The model under review builds one solid part; all positions refer to its coordinate system, in mm. A direction names the side the tool comes from. Round coordinates to 2 decimals unless told otherwise and drop trailing zeros. Write each loop counter-clockwise with the first axis right and the second up, starting at its lowest first coordinate (ties: lowest second). Pieces come first, ordered by that corner, then holes. Notation, with made-up numbers: M 33,69.5 L 79,69.5 A37 cw 79,107.5 Z; hole C -28.75,5.25 d8. An arc over 180 degrees is marked long. One line per item, written item: value. Start each with the question number.
1) Take a section at D-D, the plane x = -89. Write out the cut boundary in (y, z).
2) Take a section at C-C, the plane z = -23. Write out the cut boundary in (x, y), and give its area (3 significant figures).
3) Tool access review of faces 1 (the face through (-23.846, -107.384, -18.734)), 2 (the face through (93.2, -59.1, 25)), 3 (the face through (60, -60, 22)): name each direction out of +Z, -Z, +X, -X, +Y, -Y from which nothing blocks a thin tool from reaching the whole face with its end or side.
4) For P1, Ø6, axis at x = -78, y = -67.5, coming from the -Z side; P2, Ø2, axis at x = -14.5, z = 17, coming from the -Y side; P3, Ø6, axis at x = 50, z = 2.5, coming from the +Y side, all flat-tipped, find the tip position at first contact; note any pin that passes through.
5) Take a section at A-A, the plane x = 0. Write out the cut boundary in (y, z).
6) Mouldability with a two-part tool opening along Y and no side actions: class faces 4 (the face through (-24.93, -112.265, -6.941)), 5 (the face through (-60, 60, 22)), 6 (the face through (0, 0, -38)) as +Y half, -Y half, draft (parallel to the pull), parting line (faces both ways), or undercut.
7) Wall thickness on probe 1 along Y at (x, z) = (13.5, -15.5); probe 2 along Y at (x, z) = (0, 21.75): over which ranges is each line inside the solid? List them lowest first.
from build123d import *

# Parameters (mm, degrees)
F0_R           = 115
F1_DEPTH       = 15
F2_R           = 17.5
F3_DEPTH       = 38
F4_R           = 17.5
F5_DEPTH       = 7
F6_R           = 15.5
F7_DEPTH       = 15.5
F8_R           = 15.49999
F10_R          = 115
F10_R_2        = 110
F11_DEPTH      = 10
F11_DEPTH_BACK = 53


# Not quite as in the source:
# - a fillet or chamfer that OpenCascade refuses, or shapes differently, is made with other operations: its cross-section is extruded or revolved along the edge and cut away or added
# - a fillet or chamfer is up to 0.001 mm smaller than in the source, because OpenCascade refuses the exact size


with BuildPart() as f1:
    # F0 (on Top) → F1 (new body)
    with BuildSketch(Plane.XY):
        Circle(F0_R)
    extrude(amount=F1_DEPTH)

    # F2 (on face) → F3 (join)
    with BuildSketch(Plane(origin=(0, 0, 0), x_dir=(1, 0, 0), z_dir=(0, 0, -1))):
        Circle(F2_R)
    extrude(amount=F3_DEPTH)

    # F4 (on face) → F5 (join)
    with BuildSketch(Plane.XY.offset(15)):
        with Locations((-60, 60)):
            Circle(F4_R)
        with Locations((-60, -60)):
            Circle(F4_R)
        with Locations((60, -60)):
            Circle(F4_R)
        with Locations((60, 60)):
            Circle(F4_R)
    extrude(amount=F5_DEPTH)

    # F6 (on face) → F7 (cut)
    with BuildSketch(Plane(origin=(0, 0, 0), x_dir=(1, 0, 0), z_dir=(0, 0, -1))):
        with Locations((-60, 60)):
            Circle(F6_R)
        with Locations((-60, -60)):
            Circle(F6_R)
        with Locations((60, -60)):
            Circle(F6_R)
        with Locations((60, 60)):
            Circle(F6_R)
    extrude(amount=-F7_DEPTH, mode=Mode.SUBTRACT)

    # F8 (radius 15.5 in the source; OpenCascade refuses exactly that, so slightly less here)
    f8_edges = [f1.edges().sort_by_distance(p)[0] for p in [
        (-75.5, -60, 15.5),
        (44.5, -60, 15.5),
        (44.5, 60, 15.5),
        (-75.5, 60, 15.5),
    ]]
    fillet(f8_edges, radius=F8_R)

    # F9: fillet of radius 12 on 4 edges, made by hand

    # F9_s1 → F9_t2 (revolve, cut)
    with BuildSketch(Plane.XZ.offset(60)):
        with BuildLine():
            ThreePointArc((-42.5, 15), (-46.9279714162, 20.0995049384), (-53.4087121146, 22))
            Line((-53.4087121146, 22), (-42.5, 22))
            Line((-42.5, 22), (-42.5, 15))
        make_face()
    revolve(axis=Axis((-60, -60, 22), (0, 0, 1)), mode=Mode.SUBTRACT)

    # F9_s3 → F9_t4 (revolve, cut)
    with BuildSketch(Plane.XZ.offset(-60)):
        with BuildLine():
            ThreePointArc((-42.5, 15), (-46.9279714162, 20.0995049384), (-53.4087121146, 22))
            Line((-53.4087121146, 22), (-42.5, 22))
            Line((-42.5, 22), (-42.5, 15))
        make_face()
    revolve(axis=Axis((-60, 60, 22), (0, 0, 1)), mode=Mode.SUBTRACT)

    # F9_s5 → F9_t6 (revolve, cut)
    with BuildSketch(Plane.XZ.offset(-60)):
        with BuildLine():
            ThreePointArc((77.5, 15), (73.0720285838, 20.0995049384), (66.5912878854, 22))
            Line((66.5912878854, 22), (77.5, 22))
            Line((77.5, 22), (77.5, 15))
        make_face()
    revolve(axis=Axis((60, 60, 22), (0, 0, 1)), mode=Mode.SUBTRACT)

    # F9_s7 → F9_t8 (revolve, cut)
    with BuildSketch(Plane.XZ.offset(60)):
        with BuildLine():
            ThreePointArc((77.5, 15), (73.0720285838, 20.0995049384), (66.5912878854, 22))
            Line((66.5912878854, 22), (77.5, 22))
            Line((77.5, 22), (77.5, 15))
        make_face()
    revolve(axis=Axis((60, -60, 22), (0, 0, 1)), mode=Mode.SUBTRACT)

    # F10 (on face) → F11 (join, two sides)
    with BuildSketch(Plane.XY.offset(15)) as f11_sk:
        Circle(F10_R)
        Circle(F10_R_2, mode=Mode.SUBTRACT)
    extrude(amount=F11_DEPTH)
    extrude(f11_sk.sketch, amount=-F11_DEPTH_BACK)


solid = f1.part
Checked values:
1. outline: M -72.83,-38 L -64.65,-38 L -64.65,0 L 64.65,0 L 64.65,-38 L 72.83,-38 L 72.83,25 L 64.65,25 L 64.65,15 L -64.65,15 L -64.65,25 L -72.83,25 Z
2. outline: C 0,0 d230; C 0,0 d35; hole C 0,0 d220
2. area: 4,500 mm2
3. face 1: -Z
3. face 2: +Z, +X, -X, +Y, -Y
3. face 3: +Z
4. P1: stops at z = 0
4. P2: stops at y = -114.2
4. P3: stops at y = 104.96
5. outline: M -115,-38 L -110,-38 L -110,0 L -17.5,0 L -17.5,-38 L 17.5,-38 L 17.5,0 L 110,0 L 110,-38 L 115,-38 L 115,25 L 110,25 L 110,15 L -110,15 L -110,25 L -115,25 Z
6. face 4: parting line
6. face 5: undercut
6. face 6: draft
7. probe 1: y = -114.2 to -109.17, -11.14 to 11.14, 109.17 to 114.2
7. probe 2: y = -115 to -110, 110 to 115
